Here's how the part is built. I have some questions about the finished solid (model axes, mm). A direction names the side the tool comes from. Coordinates: 2 decimals unless noted, no trailing zeros. Order: outer loops, then holes, each group sorted by start corner. A loop starts at its lowest first (then second) coordinate and runs counter-clockwise, first axis right, second up. Notation, with made-up numbers: (51.5, 63.5) - (85.5, 63.5) arc R27 cw to (85.5, 91.5) - close; hole circle Ø4 at (25, 14). An arc over 180 degrees is marked (long way). Use CSV: the item, a comma, the result in double quotes. Start each with the question number.
Autodesk Inventor part; units mm, degrees
ref_plane "YZ Plane" through (0, 0, 0) normal (1, 0, 0) x (0, 1, 0)
ref_plane "XZ Plane" through (0, 0, 0) normal (0, 1, 0) x (-1, 0, 0)
ref_plane "XY Plane" through (0, 0, 0) normal (0, 0, 1) x (1, 0, 0)
sketch "Sketch1" plane through (0, 0, 0) normal (0, 1, 0) x (-1, 0, 0)
  circle A0 centre (0, 0) radius 1.65
  line L0 (0, 0) -> (22.8671, 0) construction
  circle A1 centre (-49.53, 0) radius 1.65
  circle A2 centre (-49.53, 0) radius 3
  line L1 (-24.765, 0) -> (-24.765, 33.4897) construction
  line L2 (0, 0) -> (0, -6.322) construction
  line L3 (-49.53, 0) -> (-44.53, 0) construction
  circle A3 centre (0, 0) radius 3
  dimension "d0" = 3.3
  dimension "d2" = 49.53
  dimension "d3" = 3.3
  dimension "d4" = 6
  dimension "d11" = 6
extrude "Extrusion1" add sketch "Sketch1" along normal blind 3
sketch "Sketch2" plane through (49.53, 0, 0) normal (0, -1, 0) x (1, 0, 0)
  line L0 (1.75, -2.2) -> (1.75, -6.339)
  line L1 (-0.25, -8.339) -> (-49.28, -8.339)
  line L2 (-51.28, -6.339) -> (-51.28, -2.2)
  line L3 (-47.78, -2.2) -> (-47.78, -3.839)
  line L4 (-46.78, -4.839) -> (-2.75, -4.839)
  line L5 (-1.75, -3.839) -> (-1.75, -2.2)
  line L6 (0, 0) -> (0, -7.7115) construction
  line L7 (1.75, -2.2) -> (-1.75, -2.2)
  line L8 (-49.53, 0) -> (-49.53, -7.2415) construction
  line L9 (-47.78, -2.2) -> (-51.28, -2.2)
  arc A0 (-47.78, -3.839) -> (-46.78, -4.839) centre (-46.78, -3.839) ccw
  arc A1 (-2.75, -4.839) -> (-1.75, -3.839) centre (-2.75, -3.839) ccw
  arc A2 (-51.28, -6.339) -> (-49.28, -8.339) centre (-49.28, -6.339) ccw
  arc A3 (-0.25, -8.339) -> (1.75, -6.339) centre (-0.25, -6.339) ccw
  point P0 (1.75, -8.339)
  point P1 (0, -2.2)
  point P2 (-49.53, -2.2)
  dimension "d14" = 6.139
  dimension "d15" = 2.2
  dimension "d16" = 3.5
  dimension "d17" = 3.5
  dimension "d18" = 2.2
  dimension "d19" = 1
  dimension "d20" = 2
extrude "Extrusion2" add sketch "Sketch2" against normal blind 3
sketch "Sketch3" plane through (49.28, 0, -8.339) normal (0, 0, -1) x (-1, 0, 0)
  arc A0 (21.6693, 0.5715) -> (22.8123, 0.5715) centre (22.2408, 0.5715) ccw
  line L0 (49.03, 0) -> (0, 0) construction
  line L1 (0, 3) -> (49.03, 3)
  line L2 (-2, 0) -> (-2, 3)
  line L3 (22.8123, 0.5715) -> (22.8123, 1.2065)
  line L4 (22.8123, 1.2065) -> (24.8123, 1.2065)
  line L5 (24.8123, 1.2065) -> (24.8123, 3)
  line L6 (21.6693, 0.5715) -> (21.6693, 1.2065)
  line L7 (21.6693, 1.2065) -> (19.6693, 1.2065)
  line L8 (19.6693, 1.2065) -> (19.6693, 3)
  line L9 (22.2408, 0.5715) -> (23.4157, 0.5715) construction
  line L10 (24.8123, 3) -> (19.6693, 3)
  point P0 (49.28, 0)
  point P1 (46.53, 3)
  point P2 (2.5, 3)
  dimension "d23" = 1.143
  dimension "d26" = 24.2408
  dimension "d27" = 2
  dimension "d28" = 2
  dimension "d29" = 0.635
  dimension "d30" = 0.635
  dimension "d31" = 2.4285
extrude "Extrusion3" add sketch "Sketch3" along normal blind 3
pattern_linear "Rectangular Pattern1" count 2 spacing 23.495 along (1, 0, 0) of "Extrusion3"
sketch "Sketch4" plane through (47.9627, 3, -8.339) normal (0, 1, 0) x (1, 0, 0)
  arc A0 (0, -5.143) -> (5.143, 0) centre (0, 0) ccw
  line L0 (5.143, 0) -> (0, 0)
  line L1 (0, 0) -> (0, -5.143)
  point P0 (-47.9627, -8.339)
extrude "Extrusion4" add sketch "Sketch4" against normal blind 3
pattern_linear "Rectangular Pattern2" count 2 spacing 5.08 along (-1, 0, 0) of "Extrusion3"
pattern_linear "Rectangular Pattern3" count 2 spacing 23.495 along (-1, 0, 0) of "Rectangular Pattern2"
sketch "Sketch6" plane through (0, 0, 0) normal (0, -1, 0) x (1, 0, 0)
  line L0 (1.0357, -8.339) -> (-4.1073, -8.339)
  line L1 (-4.1073, -8.339) -> (-1.6483, -8.339)
  line L2 (-0.2103, -8.339) -> (0.25, -8.339)
  line L3 (0.25, -8.339) -> (1.0357, -8.339)
  line L4 (1.0357, -8.339) -> (1.0357, -3.196)
  arc A0 (1.0357, -3.196) -> (-4.1073, -8.339) centre (1.0357, -8.339) ccw
  line L5 (-0.9643, -8.339) -> (0.25, -8.339)
  line L6 (-0.9643, -8.339) -> (-0.9643, -11.339)
  line L7 (1.0357, -11.339) -> (-0.9643, -11.339)
  line L8 (1.0357, -8.339) -> (1.0357, -11.339)
  line L9 (0.25, -8.339) -> (1.0357, -8.339)
  line L10 (-4.1073, -8.339) -> (-2.1073, -8.339)
  line L11 (-4.1073, -8.339) -> (-4.1073, -11.339)
  line L12 (-2.1073, -11.339) -> (-4.1073, -11.339)
  line L13 (-2.1073, -8.339) -> (-2.1073, -11.339)
  line L14 (0.25, -8.339) -> (21.9592, -8.339)
  point P0 (5.143, 0)
extrude "Extrusion5" add sketch "Sketch6" against normal blind 3 contours L0 A0 L4
sketch "Sketch7" plane through (53.1057, 3, -11.339) normal (0, 0, -1) x (-1, 0, 0)
  line L0 (3.143, -2.4285) -> (3.143, -1.7935) construction
  line L1 (3.143, -1.7935) -> (5.143, -1.7935) construction
  line L2 (5.143, -1.7935) -> (5.143, 0) construction
  line L3 (5.143, 0) -> (0, 0) construction
  line L4 (0, 0) -> (0, -1.7935) construction
  line L5 (0, -1.7935) -> (2, -1.7935) construction
  line L6 (2, -1.7935) -> (2, -2.4285) construction
  arc A0 (2, -2.4285) -> (3.143, -2.4285) centre (2.5715, -2.4285) ccw construction
  line L7 (0, -1.7935) -> (0, 0)
  line L8 (0, 0) -> (5.143, 0)
  line L9 (5.143, 0) -> (5.143, -1.7935)
  arc A1 (0, -1.7935) -> (5.143, -1.7935) centre (2.5715, -1.7935) ccw
  line L10 (5.143, -1.7935) -> (0, -1.7935) construction
  line L11 (5.143, -1.7935) -> (5.143, 0) construction
  line L12 (0, -1.7935) -> (5.143, -1.7935)
  line L13 (5.143, -1.7935) -> (5.143, -4.365)
  line L14 (5.143, -4.365) -> (0, -4.365)
  line L15 (0, -4.365) -> (0, -1.7935)
  point P0 (53.1057, -3)
  dimension "d96" = 2.5715
extrude "Extrusion6" add sketch "Sketch7" against normal blind 1.2
pattern_linear "Rectangular Pattern4" count 2 spacing 23.495 along (-1, 0, 0) of "Extrusion6"
pattern_linear "Rectangular Pattern5" count 2 spacing 28.575 along (-1, 0, 0) of "Extrusion6"
pattern_linear "Rectangular Pattern6" count 2 spacing 52.07 along (-1, 0, 0) of "Extrusion6"
sketch "Sketch9" plane through (0, 0, 0) normal (0, -1, 0) x (1, 0, 0)
  circle A0 centre (0, 0) radius 1.65
  circle A1 centre (49.53, 0) radius 1.65
  circle A2 centre (49.53, 0) radius 3.5
  arc A3 (1.75, -2.4367) -> (-1.75, -2.4367) centre (0, 0) ccw
  circle A4 centre (0, 0) radius 3.5
  point P0 (2.1649, -2.7501)
extrude "Extrusion7" [suppressed]
fillet "Fillet2" radius 2 2 edges at (1.75, 1.5, -2.4367) (47.78, 1.5, -2.4367)
fillet "Fillet3" radius 2 4 edges at (-1.75, 1.5, -2.4367) (51.28, 1.5, -2.4367) (51.28, 1.5, -4.4088) (-1.75, 1.5, -4.0158)
properties part number "HDMIPluginModuleHolder04"
Item 1: We'd pull the mould along Z, two halves only. Please class faces 1 (the cylindrical face through (51.416, 1.521, -4.294)), 2 (the flat face through (25, 3, -6)): released by +Z, released by -Z, zero draft, split by the parting line, or undercut.
Item 2: For pin 1 Ø2.5 at (x, y) = (44, 1) entering from -Z; pin 2 Ø0.5 at (x, z) = (-0.5, -9) entering from -Y; pin 3 Ø0.9 at (y, z) = (0, -9.5) entering from +X, each with a flat end and sliding along its axis, tell me the tip position at first contact or that it passes through.
Item 3: For faces 3 (the flat face through (47.963, 1.3, -10.5)), 4 (the flat face through (52, 1.206, -9)), 5 (the cylindrical face through (1.883, 1.479, -2.591)), 6 (the flat face through (29, 1.206, -9)), which set-ups out of +Z, -Z, +X, -X, +Y, -Y let a thin tool reach every point of the face, with its end or its side?
Item 4: Suppose I cut it at B-B on y = -0.65. Write out the boundary of the cut face in (x, z).
Item 5: Suppose I cut it at D-D on x = 31. Write out the boundary of the cut face in (y, z).
Item 6: Please list where these lines run through material, in increasing order: line 1 along X through (y, z) = (0.9, -10.5); line 2 along Z through (x, y) = (49.53, 1.4); line 3 along Z through (x, y) = (-1, 0.15). Write a range as from..to.
Item 7: Suppose I cut it at A-A on z = 0. Write out the boundary of the cut face in (x, y), then the cut area to 3 significant figures.
Here are the results:
1,face 1,"undercut"
1,face 2,"zero draft"
2,pin 1,"z = -8.34"
2,pin 2,"y = 1.21"
2,pin 3,"x = 51.09"
3,face 3,"-Z, +Y, -Y"
3,face 4,"+X, -Y"
3,face 5,"+Y, -Y"
3,face 6,"-Y"
4,outline,"(-4.11, -11.34) - (1.04, -11.34) - (1.04, -10.14) - (-4.11, -10.14) - close; (19.39, -11.34) - (29.61, -11.34) - (29.61, -10.14) - (19.39, -10.14) - close; (47.96, -11.34) - (53.11, -11.34) - (53.11, -10.14) - (47.96, -10.14) - close"
5,outline,"(0, -8.34) - (3, -8.34) - (3, -4.84) - (0, -4.84) - close"
6,line 1,"-4.11..1.04, 19.39..29.61, 47.96..53.11"
6,line 2,"-11.34..-1.65, 1.65..3"
6,line 3,"-11.34..-10.14, -8.34..-1.31, 1.31..2.83"
7,outline,"(-3, 0) - (-1.65, 0) - (-1.65, 3) - (-3, 3) - close; (1.65, 0) - (3, 0) - (3, 3) - (1.65, 3) - close; (46.53, 0) - (47.88, 0) - (47.88, 3) - (46.53, 3) - close; (51.18, 0) - (52.53, 0) - (52.53, 3) - (51.18, 3) - close"
7,area,"16.2 mm^2"
